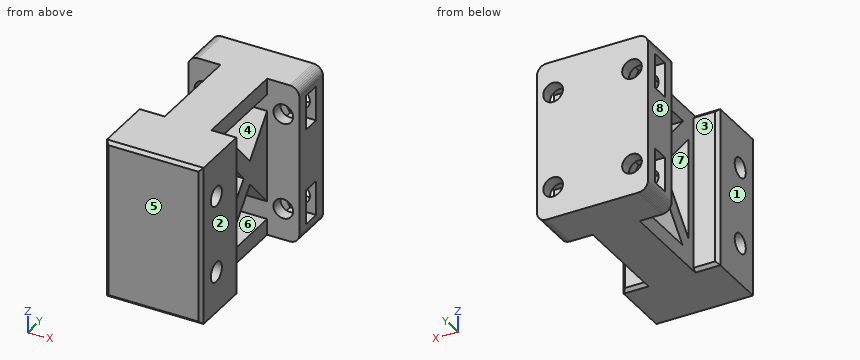
```python
from build123d import *

# Parameters (mm, degrees)
BOSS_EXTRUDE1_DEPTH = 14.49996233
SKETCH2_W           = 14.49996233
SKETCH2_H           = 39.499998092
BOSS_EXTRUDE2_DEPTH = 25.642454624
SKETCH3_W           = 14.49996233
SKETCH3_H           = 49.71832037
BOSS_EXTRUDE3_DEPTH = 4.999995232
SKETCH4_W           = 14.49996233
SKETCH4_H           = 49.71832037
BOSS_EXTRUDE4_DEPTH = 4.999995232
BOSS_EXTRUDE5_DEPTH = 13.000011444
SKETCH6_W           = 49.499988556
SKETCH6_H           = 20.018339158
BOSS_EXTRUDE6_DEPTH = 7.750034332
SKETCH7_W           = 49.499988556
SKETCH7_H           = 20.018339158
BOSS_EXTRUDE7_DEPTH = 7.750034332
CUT_EXTRUDE1_DEPTH  = 5.499958992
CUT_EXTRUDE2_START  = -13.000012
SKETCH9_R           = 3.049969673
CUT_EXTRUDE2_DEPTH  = 13.000012
CUT_EXTRUDE3_DEPTH  = 5.499958992
CUT_EXTRUDE4_REACH  = 1463.704
SKETCH11_R          = 3.049969673
CUT_EXTRUDE5_DEPTH  = 5.499958992
CUT_EXTRUDE6_REACH  = 1463.704
SKETCH13_R          = 3.049969673
CUT_EXTRUDE7_DEPTH  = 5.499958992
CUT_EXTRUDE8_REACH  = 1463.704
SKETCH15_R          = 3.049969673
SKETCH16_R          = 3.049999475
CUT_EXTRUDE9_DEPTH  = 1577.146186494
SKETCH17_R          = 3.049999475
CUT_EXTRUDE10_DEPTH = 1577.146187713
CUT_EXTRUDE15_DEPTH = 1577.006659293
CHAMFER1_SIZE2      = 0.999987125
CHAMFER1_SIZE       = 1.00004673
CHAMFER2_SIZE       = 1.00004673


with BuildPart() as part:
    # Sketch1 → Boss-Extrude1 (new body)
    with BuildSketch(Plane(origin=(652.042150497, 0, 0), x_dir=(0, -1, 0), z_dir=(-1, 0, 0))):
        Polygon((-861.958086491, 1249.692678452), (-861.958086491, 1289.192676544), (-876.510083675, 1273.185491562), (-886.033952236, 1283.933758736), (-886.033952236, 1255.276203156), (-876.557826996, 1265.699982643), (-862.374186516, 1249.692678452), align=None)
    extrude(amount=-BOSS_EXTRUDE1_DEPTH)

    # Sketch2 → Boss-Extrude2 (add)
    with BuildSketch(Plane.XZ.offset(-861.958086491)):
        with Locations((659.292131662, 1269.442677498)):
            Rectangle(SKETCH2_W, SKETCH2_H)
    extrude(amount=BOSS_EXTRUDE2_DEPTH)

    # Sketch3 → Boss-Extrude3 (add)
    with BuildSketch(Plane(origin=(0, 0, 1249.692678452), x_dir=(-1, 0, 0), z_dir=(0, 0, -1))):
        with Locations((-659.292131662, 861.174792051)):
            Rectangle(SKETCH3_W, SKETCH3_H)
    extrude(amount=BOSS_EXTRUDE3_DEPTH)

    # Sketch4 → Boss-Extrude4 (add)
    with BuildSketch(Plane.XY.offset(1289.192676544)):
        with Locations((659.292131662, 861.174792051)):
            Rectangle(SKETCH4_W, SKETCH4_H)
    extrude(amount=BOSS_EXTRUDE4_DEPTH)

    # Sketch5 → Boss-Extrude5 (add)
    with BuildSketch(Plane(origin=(0, 886.033952236, 0), x_dir=(-1, 0, 0), z_dir=(0, 1, 0))):
        Polygon((-642.744004726, 1245.764374733), (-643.113732338, 1245.394587517), (-643.54211092, 1245.094656944), (-644.016087055, 1244.873642921), (-644.521176815, 1244.738340378), (-645.04212141, 1244.69268322), (-673.542141914, 1244.69268322), (-674.06308651, 1244.738340378), (-674.56817627, 1244.873642921), (-675.042152405, 1245.094656944), (-675.470471382, 1245.394587517), (-675.840258598, 1245.764374733), (-676.140189171, 1246.19269371), (-676.361203194, 1246.666669846), (-676.496565342, 1247.171759605), (-676.542103291, 1247.692704201), (-676.542103291, 1291.192650795), (-676.496565342, 1291.71359539), (-676.361203194, 1292.21868515), (-676.140189171, 1292.692661285), (-675.840258598, 1293.121099472), (-675.470471382, 1293.490767479), (-675.042152405, 1293.790817261), (-674.56817627, 1294.011712074), (-674.06308651, 1294.147133827), (-673.542141914, 1294.192671776), (-645.04212141, 1294.192671776), (-644.521176815, 1294.147133827), (-644.016087055, 1294.011712074), (-643.54211092, 1293.790817261), (-643.113732338, 1293.490767479), (-642.744004726, 1293.121099472), (-642.444074154, 1292.692661285), (-642.223060131, 1292.21868515), (-642.087697983, 1291.71359539), (-642.04210043, 1291.192650795), (-642.04210043, 1247.692704201), (-642.087697983, 1247.171759605), (-642.223060131, 1246.666669846), (-642.444074154, 1246.19269371), align=None)
    extrude(amount=BOSS_EXTRUDE5_DEPTH)

    # Sketch6 → Boss-Extrude6 (add)
    with BuildSketch(Plane.ZY.offset(-652.042150497)):
        with Locations((1269.442677498, 846.324801445)):
            Rectangle(SKETCH6_W, SKETCH6_H)
    extrude(amount=BOSS_EXTRUDE6_DEPTH)

    # Sketch7 → Boss-Extrude7 (add)
    with BuildSketch(Plane(origin=(666.542112827, 0, 0), x_dir=(0, 0, -1), z_dir=(1, 0, 0))):
        with Locations((-1269.442677498, 846.324801445)):
            Rectangle(SKETCH7_W, SKETCH7_H)
    extrude(amount=BOSS_EXTRUDE7_DEPTH)

    # Sketch8 → Cut-Extrude1 (cut)
    with BuildSketch(Plane.XZ.offset(-889.783978462)):
        Polygon((676.542103291, 1259.846687317), (668.422102928, 1259.846687317), (665.302097797, 1254.442691803), (668.422102928, 1249.038696289), (676.542103291, 1249.038696289), align=None)
    extrude(amount=-CUT_EXTRUDE1_DEPTH, mode=Mode.SUBTRACT)

    # Sketch9 → Cut-Extrude2 (cut)
    with BuildSketch(Plane(origin=(0, 899.03396368, 0), x_dir=(-1, 0, 0), z_dir=(0, 1, 0)).offset(CUT_EXTRUDE2_START)):
        with Locations(Location((-671.542108059, 1254.442691803, 0), (0, 0, 90))):
            Circle(SKETCH9_R)
    extrude(amount=CUT_EXTRUDE2_DEPTH, mode=Mode.SUBTRACT)

    # Sketch10 → Cut-Extrude3 (cut)
    with BuildSketch(Plane.XZ.offset(-889.783978462)):
        Polygon((642.04210043, 1249.038696289), (650.162100792, 1249.038696289), (653.282105923, 1254.442691803), (650.162100792, 1259.846687317), (642.04210043, 1259.846687317), align=None)
    extrude(amount=-CUT_EXTRUDE3_DEPTH, mode=Mode.SUBTRACT)

    # Cut-Extrude4: up to this face of the body (flat: up to its plane)
    cut_extrude4_end = Plane(part.part.faces().sort_by_distance((643.088277536, 886.033952236, 1246.324624689))[0])
    # Sketch11 → Cut-Extrude4 (cut, up to the picked face)
    with BuildSketch(Plane(origin=(0, 899.03396368, 0), x_dir=(-1, 0, 0), z_dir=(0, 1, 0)), mode=Mode.PRIVATE) as cut_extrude4_sk1:
        with Locations(Location((-647.042095661, 1254.442691803, 0), (0, 0, 90))):
            Circle(SKETCH11_R)
    cut_extrude4_tool1 = split(extrude(cut_extrude4_sk1.sketch, amount=-CUT_EXTRUDE4_REACH, mode=Mode.PRIVATE), bisect_by=cut_extrude4_end, keep=Keep.BOTH, mode=Mode.PRIVATE)
    add(cut_extrude4_tool1.solids().sort_by(Axis((647.042096, 899.033964, 1254.442692), (0, -1, 0)))[0], mode=Mode.SUBTRACT)

    # Sketch12 → Cut-Extrude5 (cut)
    with BuildSketch(Plane.XZ.offset(-889.783978462)):
        Polygon((642.04210043, 1279.038667679), (650.162100792, 1279.038667679), (653.282105923, 1284.442663193), (650.162100792, 1289.846658707), (642.04210043, 1289.846658707), align=None)
    extrude(amount=-CUT_EXTRUDE5_DEPTH, mode=Mode.SUBTRACT)

    # Cut-Extrude6: up to this face of the body (flat: up to its plane)
    cut_extrude6_end = Plane(part.part.faces().sort_by_distance((643.088277536, 886.033952236, 1246.324624689))[0])
    # Sketch13 → Cut-Extrude6 (cut, up to the picked face)
    with BuildSketch(Plane(origin=(0, 899.03396368, 0), x_dir=(-1, 0, 0), z_dir=(0, 1, 0)), mode=Mode.PRIVATE) as cut_extrude6_sk1:
        with Locations(Location((-647.042095661, 1284.442663193, 0), (0, 0, 90))):
            Circle(SKETCH13_R)
    cut_extrude6_tool1 = split(extrude(cut_extrude6_sk1.sketch, amount=-CUT_EXTRUDE6_REACH, mode=Mode.PRIVATE), bisect_by=cut_extrude6_end, keep=Keep.BOTH, mode=Mode.PRIVATE)
    add(cut_extrude6_tool1.solids().sort_by(Axis((647.042096, 899.033964, 1284.442663), (0, -1, 0)))[0], mode=Mode.SUBTRACT)

    # Sketch14 → Cut-Extrude7 (cut)
    with BuildSketch(Plane.XZ.offset(-889.783978462)):
        Polygon((676.542103291, 1289.846658707), (668.422102928, 1289.846658707), (665.302097797, 1284.442663193), (668.422102928, 1279.038667679), (676.542103291, 1279.038667679), align=None)
    extrude(amount=-CUT_EXTRUDE7_DEPTH, mode=Mode.SUBTRACT)

    # Cut-Extrude8: up to this face of the body (flat: up to its plane)
    cut_extrude8_end = Plane(part.part.faces().sort_by_distance((643.088277536, 886.033952236, 1246.324624689))[0])
    # Sketch15 → Cut-Extrude8 (cut, up to the picked face)
    with BuildSketch(Plane(origin=(0, 899.03396368, 0), x_dir=(-1, 0, 0), z_dir=(0, 1, 0)), mode=Mode.PRIVATE) as cut_extrude8_sk1:
        with Locations(Location((-671.542108059, 1284.442663193, 0), (0, 0, 90))):
            Circle(SKETCH15_R)
    cut_extrude8_tool1 = split(extrude(cut_extrude8_sk1.sketch, amount=-CUT_EXTRUDE8_REACH, mode=Mode.PRIVATE), bisect_by=cut_extrude8_end, keep=Keep.BOTH, mode=Mode.PRIVATE)
    add(cut_extrude8_tool1.solids().sort_by(Axis((671.542108, 899.033964, 1284.442663), (0, -1, 0)))[0], mode=Mode.SUBTRACT)

    # Sketch16 → Cut-Extrude9 (cut, through all)
    with BuildSketch(Plane.ZY.offset(-644.292116165)):
        with Locations((1281.442642212, 844.333976507)):
            Circle(SKETCH16_R)
    extrude(amount=-CUT_EXTRUDE9_DEPTH, mode=Mode.SUBTRACT)

    # Sketch17 → Cut-Extrude10 (cut, through all)
    with BuildSketch(Plane(origin=(674.29214716, 0, 0), x_dir=(0, 0, -1), z_dir=(1, 0, 0))):
        with Locations((-1257.442712784, 844.333976507)):
            Circle(SKETCH17_R)
    extrude(amount=-CUT_EXTRUDE10_DEPTH, mode=Mode.SUBTRACT)

    # Sketch22 → Cut-Extrude15 (cut, through all)
    with BuildSketch(Plane(origin=(666.542112827, 0, 0), x_dir=(0, 0, -1), z_dir=(1, 0, 0))):
        Polygon((-1253.462314606, 859.033942223), (-1269.421219826, 873.174786568), (-1284.976124763, 859.033942223), align=None)
    extrude(amount=-CUT_EXTRUDE15_DEPTH, mode=Mode.SUBTRACT)

    # Chamfer1
    chamfer1_edges = [part.edges().sort_by_distance(p)[0] for p in [
        (648.167133331, 856.333971024, 1294.192671776),
        (648.167133331, 856.333971024, 1244.69268322),
        (644.292116165, 856.333971024, 1269.442677498),
        (670.417129993, 856.333971024, 1244.69268322),
        (670.417129993, 856.333971024, 1294.192671776),
        (674.29214716, 856.333971024, 1269.442677498),
    ]]
    chamfer(chamfer1_edges, length=CHAMFER1_SIZE, length2=CHAMFER1_SIZE2)

    # Chamfer2
    chamfer2_edges = [part.edges().sort_by_distance(p)[0] for p in [
        (644.292116165, 836.315631866, 1269.442677498),
        (674.29214716, 836.315631866, 1269.442677498),
        (659.292131662, 836.315631866, 1244.69268322),
        (659.292131662, 836.315631866, 1294.192671776),
    ]]
    chamfer(chamfer2_edges, length=CHAMFER2_SIZE)


solid = part.part
```
Build history of the part. All positions in model axes, mm. Face numbers are marked on the shaded views. A direction names the side the tool comes from. Round coordinates to 2 decimals unless told otherwise and drop trailing zeros. Loops run counter-clockwise (first coordinate to the right, second up) from the corner with the lowest first, then second, coordinate; pieces in that order, holes last.
Item 1: Saw through at C-C (x = 667.5). List the corners of the cut face in (y, z).
Item 2: Pin check, flat tips, straight feed: P1, Ø5.5, axis at y = 845, z = 1264, coming from the +X side; P2, Ø5, axis at y = 867.5, z = 1259, coming from the -X side; P3, Ø3.5, axis at x = 671.54, z = 1284.44, coming from the +Y side. Stop position of each tip, or through.
Item 3: Saw through at B-B (y = 867.5). List the corners of the cut face in (x, z).
Item 4: Which spindle directions (+Z, -Z, +X, -X, +Y, -Y) get a long thin tool onto all of the face, cutting with end or side? Do the marked faces 1, 2, 3 and 4. Say none if no direction does.
Item 5: Two-plate mould, pull along Y, no slides. Class the marked faces 5, 6, 7 and 8: released by +Y, released by -Y, zero draft, split by the parting line, or undercut.
Item 6: Drill centre lines: line 1 along Z through (x, y) = (672.5, 891); line 2 along Z through (x, y) = (644.5, 890); line 3 along Y through (x, z) = (653, 1281.5). Where is each one in solid material? Low to high.
Item 7: Saw through at D-D (y = 875). List the corners of the cut face in (x, z).
Item 8: Saw through at A-A (z = 1277.5). List the corners of the cut face in (x, y), then the cut area to 3 significant figures.
Worked answers:
1. outline: (836.32, 1245.69) - (837.32, 1244.69) - (855.33, 1244.69) - (856.33, 1245.69) - (856.33, 1293.19) - (855.33, 1294.19) - (837.32, 1294.19) - (836.32, 1293.19) - close; (886.03, 1244.69) - (899.03, 1244.69) - (899.03, 1294.19) - (886.03, 1294.19) - close; hole circle Ø6.1 at (844.33, 1257.44); hole circle Ø6.1 at (844.33, 1281.44); hole (889.78, 1250.64) - (895.28, 1250.64) - (895.28, 1258.25) - (889.78, 1258.25) - close; hole (889.78, 1280.64) - (895.28, 1280.64) - (895.28, 1288.25) - (889.78, 1288.25) - close
2. P1: stops at x = 674.29
2. P2: stops at x = 652.04
2. P3: stops at y = 856.33
3. outline: (652.04, 1244.69) - (666.54, 1244.69) - (666.54, 1249.69) - (652.04, 1249.69) - close; (652.04, 1255.48) - (666.54, 1255.48) - (666.54, 1263.02) - (652.04, 1263.02) - close; (652.04, 1275.66) - (666.54, 1275.66) - (666.54, 1283.1) - (652.04, 1283.1) - close; (652.04, 1289.19) - (666.54, 1289.19) - (666.54, 1294.19) - (652.04, 1294.19) - close
4. face 1: +Z, -Z, -X, -Y
4. face 2: +Z, -Z, +X, -Y
4. face 3: +Z, -Z, -X
4. face 4: +X, -X
5. face 5: released by -Y
5. face 6: undercut
5. face 7: undercut
5. face 8: zero draft
6. line 1: z = 1244.69 to 1249.04, 1259.85 to 1279.04, 1289.85 to 1294.19
6. line 2: z = 1244.74 to 1249.04, 1259.85 to 1279.04, 1289.85 to 1294.14
6. line 3: y = 836.32 to 841.28, 847.38 to 859.03, 862.19 to 868.95, 883.88 to 899.03
7. outline: (652.04, 1244.69) - (666.54, 1244.69) - (666.54, 1249.69) - (652.04, 1249.69) - close; (652.04, 1263.94) - (666.54, 1263.94) - (666.54, 1274.85) - (652.04, 1274.85) - close; (652.04, 1289.19) - (666.54, 1289.19) - (666.54, 1294.19) - (652.04, 1294.19) - close
8. outline: (642.04, 886.03) - (652.04, 886.03) - (652.04, 880.33) - (666.54, 880.33) - (666.54, 886.03) - (676.54, 886.03) - (676.54, 899.03) - (642.04, 899.03) - close; (644.29, 837.32) - (645.29, 836.32) - (673.29, 836.32) - (674.29, 837.32) - (674.29, 855.33) - (673.29, 856.33) - (666.54, 856.33) - (666.54, 859.03) - (652.04, 859.03) - (652.04, 856.33) - (645.29, 856.33) - (644.29, 855.33) - close; (652.04, 865.83) - (666.54, 865.83) - (666.54, 872.59) - (652.04, 872.59) - close
8. area: 1,270 mm2
